Part print with two shaded views. Sizes in mm from the minimum x, y, z corner. Give positions to 0.01 mm unless a question says otherwise; leave off trailing zeros. Order: outer loops, then holes, each group sorted by start corner. A loop starts at its lowest first (then second) coordinate and runs counter-clockwise, first axis right, second up. Notation, with made-up numbers: M 59.5,28 L 65.5,28 A22 ccw 65.5,34 Z; hole C 81.5,84.5 d1. An arc over 180 degrees is marked long. Return JSON: item names as keys, results as strings.
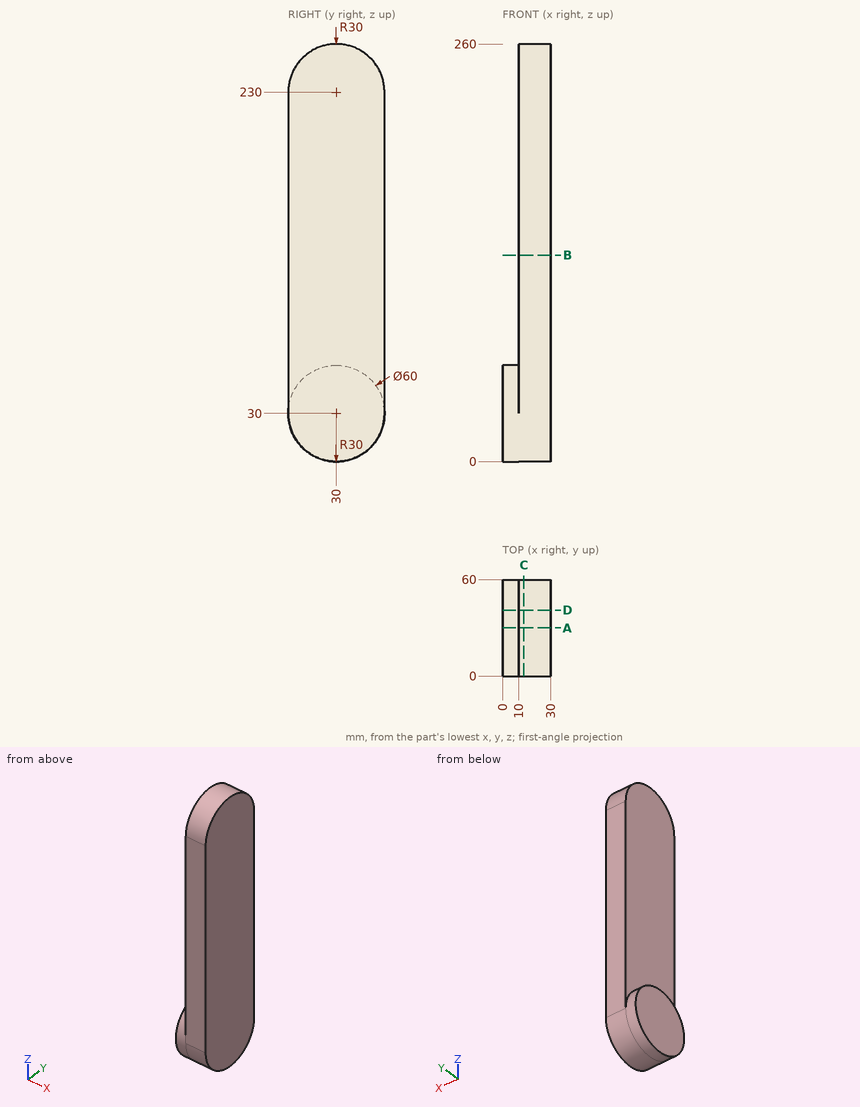
Q1. Band-saw the part on D-D (y = 41). Give the cut face in (x, z), then the cut area to 3 significant figures.
Established:
{"outline": "M 0,2.09 L 30,2.09 L 30,257.91 L 10,257.91 L 10,57.91 L 0,57.91 Z", "area": "5,670 mm²"}
Q2. Probe line 1 along X through (y, z) = (36, 97.5); line 2 along Z through (x, y) = (4.5, 29.5); line 3 along Z through (x, y) = (19.5, 34). List the from-to ranges inside material, lowest first.
Established:
{"line 1": "x = 10 to 30", "line 2": "z = 0 to 60", "line 3": "z = 0.27 to 259.73"}
Q3. Pin check, flat tips, straight feed: pin 1 (1 mm diameter, centred on x = 17, y = 20, fed in from +Z); pin 2 (10 mm diameter, centred on x = 17, y = 46.5, fed in from -Z); pin 3 (1 mm diameter, centred on y = 16, z = 204.5, fed in from -X); pin 4 (6 mm diameter, centred on x = 4.5, z = 63.5, fed in from +Y). Stop position of each tip, or through.
Established:
{"pin 1": "stops at z = 258.46", "pin 2": "stops at z = 2.29", "pin 3": "stops at x = 10", "pin 4": "passes through"}
Q4. Band-saw the part on C-C (x = 13.25). Give the cut face in (y, z), then the cut area to 3 significant figures.
Established:
{"outline": "M 0,30 A30 ccw 60,30 L 60,230 A30 ccw 0,230 Z", "area": "14,800 mm²"}
Q5. Band-saw the part on B-B (z = 128.5). Give the cut face in (x, y), then the cut area to 3 significant figures.
Established:
{"outline": "M 10,0 L 30,0 L 30,60 L 10,60 Z", "area": "1,200 mm²"}
Q6. Band-saw the part on A-A (y = 30). Give the cut face in (x, z), then the cut area to 3 significant figures.
Established:
{"outline": "M 0,0 L 30,0 L 30,260 L 10,260 L 10,60 L 0,60 Z", "area": "5,800 mm²"}
